Autodesk Inventor part; units mm, degrees
ref_plane "YZ Plane" through (0, 0, 0) normal (1, 0, 0) x (0, 1, 0)
ref_plane "XZ Plane" through (0, 0, 0) normal (0, 1, 0) x (-1, 0, 0)
ref_plane "XY Plane" through (0, 0, 0) normal (0, 0, 1) x (1, 0, 0)
sketch "Sketch1" plane through (0, 0, 0) normal (0, 0, 1) x (1, 0, 0)
  circle A0 centre (0, 0) radius 20
  circle A1 centre (0, -120) radius 11
  circle A2 centre (-235, -320) radius 11
  circle A3 centre (235, -320) radius 11
  arc A4 (233.6625, -350) -> (260.9808, -293.1206) centre (233.6625, -315) ccw
  line L0 (260.9808, -293.1206) -> (60, 0)
  line L1 (0, 0) -> (0, -429.6945)
  arc A5 (-260.9808, -293.1206) -> (-233.6625, -350) centre (-233.6625, -315) ccw
  line L2 (-260.9808, -293.1206) -> (-60, 0)
  spline S0 degree 2 poles (-60, 0) (0.0011, 80.0234) (60, 0) knots 0 0 0 1 1 1
  line L3 (0, -150) -> (70, -150)
  line L4 (-80, -240) -> (-80, -160)
  line L5 (-70, -150) -> (0, -150)
  line L6 (-80, -160) -> (-70, -150)
  line L7 (80, -160) -> (70, -150)
  line L8 (-80, -160) -> (-80, -350)
  line L9 (80, -160) -> (80, -350)
  line L10 (-233.6625, -350) -> (-80, -350)
  line L11 (80, -350) -> (233.6625, -350)
  circle A6 centre (-110, -320) radius 11
  circle A7 centre (110, -320) radius 11
  point P0 (0.0008, 40.0117)
  point P1 (80, -150)
  point P2 (60, -250)
  point P3 (-80, -150)
  dimension "d0" = 40
  dimension "d1" = 22
  dimension "d3" = 22
  dimension "d4" = 22
  dimension "d5" = 120
  dimension "d9" = 35
  dimension "d14" = 60
  dimension "d15" = 60
  dimension "d16" = 80
  dimension "d19" = 10
  dimension "d20" = 10
  dimension "d21" = 10
  dimension "d22" = 10
  dimension "d27" = 30
  dimension "d30" = 22
  dimension "d31" = 22
  dimension "d32" = 30
  dimension "d33" = 30
  dimension "d36" = 160
extrude "Extrusion2" add sketch "Sketch1" along normal mid plane 22.22
properties part number "Corpo_Suporte_4_Cabos_Modelo3"
Can you work these out from the model? Positions are in its coordinate system, mm. A direction names the side the tool comes from. Give positions to 0.01 mm unless a question says otherwise; leave off trailing zeros. Order: outer loops, then holes, each group sorted by start corner. A loop starts at its lowest first (then second) coordinate and runs counter-clockwise, first axis right, second up. Notation, with made-up numbers: (-15.5, 36.25) - (4.5, 36.25) arc R31 cw to (4.5, 74.25) - close; hole circle Ø3 at (11.5, 36). An arc over 180 degrees is marked (long way). Use a Markdown table: item, result. Add a question column.
Q1. If we section it at D-D on x = 0: Count the separate pieces of the cut face and the enclosed holes in it, plus the area to 3 significant figures.
Q2. If we section it at C-C on y = -320: Write out the boundary of the cut face in (x, z).
Q3. If we section it at B-B on x = -110: Write out the boundary of the cut face in (y, z), plus the area to 3 significant figures.
Q4. I'm going to push flat-ended pins straight in: pin 1 (11 mm diameter, centred on y = -281, z = 0, fed in from -X); pin 2 (17.5 mm diameter, centred on x = 235, y = -320, fed in from +Z); pin 3 (10 mm diameter, centred on y = -308, z = -1.5, fed in from -X); pin 4 (3 mm diameter, centred on y = -10.5, z = 3.5, fed in from -X). Where does each tip first touch, or does it pass through?
Q5. On a 3-axis mill with a long thin cutter (end or side, diameter ignored), from which of +Z, -Z, +X, -X, +Y, -Y can I reach the whole of each face in a straight line? I mean faces 4 (the flat face through (-158, -350, 0)), 5 (the flat face through (-1, -150, 0)). Say none if no direction works.
Q6. If we mould it in two halves opening along X, with no side actions, what happens to faces 1 (the flat face through (-161.897, -148.612, -0.156)), 2 (the flat face through (75, -155, 0)), 3 (the flat face through (19, -134, -11.11))? For each: released by +X, released by -X, zero draft, split by the parting line, or undercut.
Q7. If we section it at A-A on y = -174: Write out the boundary of the cut face in (x, z).
Q8. Please list where these lines run through material, in increasing order: line 1 along Y through (x, z) = (0, 4.25); line 2 along X through (y, z) = (-188, 10.25); line 3 along X through (y, z) = (0, 3).
Answers follow:
| question | item | result |
|---|---|---|
| 1 | separate pieces | 3 |
| 1 | enclosed holes | 0 |
| 1 | area | 2,840 mm^2 |
| 2 | outline | (-268.3, -11.11) - (-246, -11.11) - (-246, 11.11) - (-268.3, 11.11) - close; (-224, -11.11) - (-121, -11.11) - (-121, 11.11) - (-224, 11.11) - close; (-99, -11.11) - (-80, -11.11) - (-80, 11.11) - (-99, 11.11) - close; (80, -11.11) - (99, -11.11) - (99, 11.11) - (80, 11.11) - close; (121, -11.11) - (224, -11.11) - (224, 11.11) - (121, 11.11) - close; (246, -11.11) - (268.3, -11.11) - (268.3, 11.11) - (246, 11.11) - close |
| 3 | outline | (-350, -11.11) - (-331, -11.11) - (-331, 11.11) - (-350, 11.11) - close; (-309, -11.11) - (-72.92, -11.11) - (-72.92, 11.11) - (-309, 11.11) - close |
| 3 | area | 5,670 mm^2 |
| 4 | pin 1 | stops at x = -256.44 |
| 4 | pin 2 | passes through |
| 4 | pin 3 | stops at x = -268.61 |
| 4 | pin 4 | stops at x = -68.23 |
| 5 | face 4 | +Z, -Z, +X, -X, -Y |
| 5 | face 5 | +Z, -Z, -Y |
| 6 | face 1 | released by -X |
| 6 | face 2 | undercut |
| 6 | face 3 | zero draft |
| 7 | outline | (-179.3, -11.11) - (-80, -11.11) - (-80, 11.11) - (-179.3, 11.11) - close; (80, -11.11) - (179.3, -11.11) - (179.3, 11.11) - (80, 11.11) - close |
| 8 | line 1 | y = -150 to -131, -109 to -20, 20 to 40.01 |
| 8 | line 2 | x = -188.9 to -80, 80 to 188.9 |
| 8 | line 3 | x = -60 to -20, 20 to 60 |
